Here's how the part is built. I have some questions about the finished solid (model axes, mm). A direction names the side the tool comes from. Round coordinates to 2 decimals unless told otherwise and drop trailing zeros. Order: outer loops, then holes, each group sorted by start corner. A loop starts at its lowest first (then second) coordinate and runs counter-clockwise, first axis right, second up. Notation, with made-up numbers: M 74,-26.75 L 79,-26.75 A17 cw 79,-13.75 Z; hole C 79,29.25 d11. An arc over 180 degrees is marked long. Use one line per item in the form item = value. Start each with the question number.
Autodesk Fusion 360 part; units mm, degrees
sketch "スケッチ1" plane through (0, 0, 0) normal (0, 0, 1) x (1, 0, 0)
  line L0 (55, 0) -> (45, 0)
  line L1 (45, 0) -> (0, 45)
  line L2 (0, 45) -> (0, 55)
  line L3 (0, 55) -> (40, 95)
  line L4 (40, 95) -> (95, 40)
  line L5 (95, 40) -> (55, 0)
extrude "押し出し1" add sketch "スケッチ1" along normal blind 5
sketch "スケッチ2" plane through (0, 0, 5) normal (0, 0, 1) x (-1, 0, 0)
  line L0 (-95, -40) -> (-40, -95)
  line L1 (-40, -95) -> (0, -55)
  line L2 (0, -55) -> (0, -45)
  line L3 (0, -45) -> (-45, 0)
  line L4 (-45, 0) -> (-55, 0)
  line L5 (-55, 0) -> (-95, -40)
  line L6 (-55, -10) -> (-80, -35)
  line L7 (-80, -45) -> (-45, -80)
  line L8 (-35, -80) -> (-10, -55)
  line L9 (-10, -55) -> (-55, -10)
  line L10 (-35, -80) -> (-45, -80)
  line L11 (-80, -45) -> (-80, -35)
  line L12 (-62.5, -62.5) -> (-32.5, -32.5)
  circle A0 centre (-47.5, -47.5) radius 21.225
  circle A1 centre (-40.7825, -40.7825) radius 1.5
  circle A2 centre (-56.3388, -38.6612) radius 1.5
  circle A3 centre (-54.2175, -54.2175) radius 1.5
  circle A4 centre (-38.6612, -56.3388) radius 1.5
  line L13 (-38.6612, -56.3388) -> (-56.3388, -38.6612)
  circle A5 centre (-47.5, -47.5) radius 4
  point P0 (-47.5, -47.5)
  dimension "d4" = 3
  dimension "d11" = 19
  dimension "d12" = 12.5
  dimension "d13" = 12.5
  dimension "d14" = 3
  dimension "d15" = 3
  dimension "d16" = 3
  dimension "d17" = 8
sketch "スケッチ3" plane through (0, 0, 5) normal (0, 0, 1) x (-1, 0, 0)
  circle A0 centre (-5, -52) radius 1.5
  circle A1 centre (-52, -5) radius 1.5
  circle A2 centre (-40, -87) radius 1.5
  circle A3 centre (-87, -40) radius 1.5
extrude "押し出し2" cut sketch "スケッチ3" sketch "スケッチ2" against normal blind 5 of sketch 2 contours A2 | A4 | L12 A1 | L12 A1 | L12 A3 | L12 A3
sketch "スケッチ4" plane through (0, 0, 0) normal (0, 0, -1) x (1, 0, 0)
  line L0 (40, -95) -> (95, -40)
  line L1 (95, -40) -> (55, 0)
  line L2 (55, 0) -> (45, 0)
  line L3 (45, 0) -> (0, -45)
  line L4 (0, -45) -> (0, -55)
  line L5 (0, -55) -> (40, -95)
  circle A0 centre (38.6612, -56.3388) radius 1.5
  circle A1 centre (54.2175, -54.2175) radius 1.5
  circle A2 centre (87, -40) radius 1.5
  circle A3 centre (40, -87) radius 1.5
  circle A4 centre (52, -5) radius 1.5
  circle A5 centre (5, -52) radius 1.5
  circle A6 centre (40.7825, -40.7825) radius 1.5
  circle A7 centre (56.3388, -38.6612) radius 1.5
  line L6 (85, -50) -> (80, -45)
  line L7 (80, -45) -> (45, -80)
  line L8 (45, -80) -> (50, -85)
  line L9 (85, -50) -> (50, -85)
extrude "押し出し3" cut sketch "スケッチ4" against normal blind 5 contours L0 L6 L7 L8 L9
extrude "押し出し4" cut sketch "スケッチ2" against normal blind 12 contours L12 L13 A5 | L12 L13 A5 | L12 L13 A5 | L12 L13 A5
1) Will these pins go through, and if not, where does the flat tip stop? pin 1 Ø2 at (y, z) = (66.5, 2.5) entering from -X; pin 2 Ø3.5 at (x, y) = (40.78, 40.78) entering from -Z; pin 3 Ø3 at (y, z) = (63, 3.5) entering from +X.
2) If we section it at B-B on y = 87: Write out the boundary of the cut face in (x, z).
3) If we section it at D-D on z = 0.75: Give the number of separate pieces and of enclosed holes in the cut face, then the cut area to 3 significant figures.
4) If we section it at A-A on x = 47.5: Write out the boundary of the cut face in (y, z), then the cut area to 4 significant figures.
5) If I drill on line 1 (X direction, y = 55.5, z = 2.7); line 2 (X direction, y = 40.5, z = 1.8); line 3 (X direction, y = 5, z = 3.5), over which ranges is the centre line in solid material (lowest first)?
6) On a 3-axis mill with a long thin cutter (end or side, diameter ignored), from which of +Z, -Z, +X, -X, +Y, -Y can I reach the whole of each face in a straight line? I mean faces 1 (the flat face through (47, 82, 2)), 2 (the cylindrical face through (40.195, 85.513, 2.535)), 3 (the flat face through (83, 48, 2)). Say none if no direction works.
7) If we mould it in two halves opening along Y, with no side actions, what happens to faces 4 (the flat face through (23, 22, 2)), 5 (the flat face through (36, 48, 5)), 6 (the cylindrical face through (56.664, 40.126, 2.535))? For each: +Y half, -Y half, draft (parallel to the pull), parting line (faces both ways), or undercut.
Completed:
q1.pin_1 = 10.5
q1.pin_2 = 0
q1.pin_3 = 63.5
q2.outline = M 32,0 L 38.5,0 L 38.5,5 L 32,5 Z; M 41.5,0 L 48,0 L 48,5 L 41.5,5 Z
q3.separate_pieces = 1
q3.enclosed_holes = 9
q3.area = 4,440 mm²
q4.outline = M 0,0 L 43.5,0 L 43.5,5 L 0,5 Z; M 51.5,0 L 77.5,0 L 77.5,5 L 51.5,5 Z; M 82.5,0 L 87.5,0 L 87.5,5 L 82.5,5 Z
q4.area = 372.5 mm²
q5.line_1 = 0.5 to 37.42, 39.9 to 53.44, 55 to 69.5
q5.line_2 = 4.5 to 39.31, 42.26 to 85.59, 88.41 to 94.5
q5.line_3 = 40 to 50.5, 53.5 to 60
q6.face_1 = +Z, -Z, +X
q6.face_2 = +Z, -Z
q6.face_3 = +Z, -Z, +Y
q7.face_4 = -Y half
q7.face_5 = draft
q7.face_6 = undercut
